Geometry: final body of the model. Coordinates: model frame, mm. Give positions to 0.01 mm unless a question says otherwise; leave off trailing zeros. Write each loop counter-clockwise with the first axis right and the second up, starting at its lowest first coordinate (ties: lowest second). Pieces come first, ordered by that corner, then holes.
Q1. Draft query along Y for faces 1 (the face through (230.495, 14.758, 19.367)), 2 (the face through (0, 67, 20)), 3 (the face through (4.51, 4.28, 19.72)), 4 (the face through (210.974, 29.257, 24.79)). Return one class per face: pulls with the +Y half, pulls with the -Y half, needs draft (parallel to the pull), parting line crosses it, or undercut.
Q2. Pin query (flat end, axial travel): pin 1 (5.5 mm diameter, centred on x = 226, y = 15, fed in from +Z); pin 2 (9 mm diameter, centred on x = 224, y = 121, fed in from +Z); pin 3 (4.5 mm diameter, centred on x = 160, y = 73.79, fed in from +Z). Return the tip coordinate at first contact, or that it passes through.
Q3. Cut plane B-B on z = 22. Count the separate pieces of the cut face and the enclosed holes in it, plus the area to 3 significant figures.
Q4. Cut plane A-A on y = 43.5. Return the cut outline in (x, z).
Q5. Line query: L1, parallel to X at y = 78, z = 11; L2, parallel to Y at x = 80, z = 26.25; L3, parallel to Y at x = 40.5, z = 30. Output: solid intervals per line, ascending.
```python
from build123d import *

# Parameters (mm, degrees)
SKETCH_1_R                   = 5.5
EXTRUDE_1_DEPTH              = 40
EXTRUDE_2_DEPTH              = 10
EXTRUDE_3_DEPTH              = 20
HOLE_WIZARD_M6_3_D           = 5
HOLE_WIZARD_M6_3_DEPTH       = 15
HOLE_WIZARD_M6_3_CSINK_D     = 8
HOLE_WIZARD_M6_3_CSINK_ANGLE = 90
HOLE_WIZARD_M6_3_TIP         = 1.502151548
SKETCH_9_R                   = 9
CUT_EXTRUDE_1_DEPTH          = 11
CHAMFER_2_SIZE               = 1
CHAMFER_3_SIZE               = 1


with BuildPart() as part:
    # 草图1 → 凸台-拉伸1 (new body)
    with BuildSketch(Plane.XY):
        with BuildLine():
            Line((0, 15), (0, 120))
            ThreePointArc((0, 120), (4.393398282, 130.606601718), (15, 135))
            Line((15, 135), (225, 135))
            ThreePointArc((225, 135), (235.606601718, 130.606601718), (240, 120))
            Line((240, 120), (240, 15))
            ThreePointArc((240, 15), (235.606601718, 4.393398282), (225, 0))
            Line((225, 0), (15, 0))
            ThreePointArc((15, 0), (4.393398282, 4.393398282), (0, 15))
        make_face()
        with Locations((225, 120)):
            Circle(SKETCH_1_R, mode=Mode.SUBTRACT)
        with Locations(Location((225, 15, 0), (0, 0, 180))):
            Circle(SKETCH_1_R, mode=Mode.SUBTRACT)
        with Locations((15, 15)):
            Circle(SKETCH_1_R, mode=Mode.SUBTRACT)
        with Locations(Location((15, 120, 0), (0, 0, 180))):
            Circle(SKETCH_1_R, mode=Mode.SUBTRACT)
        with BuildLine():
            Line((15, 39.494897428), (15, 95.505102572))
            ThreePointArc((15, 95.505102572), (16.127016654, 98.667380232), (19, 100.404082058))
            ThreePointArc((19, 100.404082058), (29.142135624, 105.857864376), (34.595917942, 116))
            ThreePointArc((34.595917942, 116), (36.332619768, 118.872983346), (39.494897428, 120))
            Line((39.494897428, 120), (200.505102572, 120))
            ThreePointArc((200.505102572, 120), (203.667380232, 118.872983346), (205.404082058, 116))
            ThreePointArc((205.404082058, 116), (210.857864376, 105.857864376), (221, 100.404082058))
            ThreePointArc((221, 100.404082058), (223.872983346, 98.667380232), (225, 95.505102572))
            Line((225, 95.505102572), (225, 39.494897428))
            ThreePointArc((225, 39.494897428), (223.872983346, 36.332619768), (221, 34.595917942))
            ThreePointArc((221, 34.595917942), (210.857864376, 29.142135624), (205.404082058, 19))
            ThreePointArc((205.404082058, 19), (203.667380232, 16.127016654), (200.505102572, 15))
            Line((200.505102572, 15), (39.494897428, 15))
            ThreePointArc((39.494897428, 15), (36.332619768, 16.127016654), (34.595917942, 19))
            ThreePointArc((34.595917942, 19), (29.142135624, 29.142135624), (19, 34.595917942))
            ThreePointArc((19, 34.595917942), (16.127016654, 36.332619768), (15, 39.494897428))
        make_face(mode=Mode.SUBTRACT)
    extrude(amount=EXTRUDE_1_DEPTH)

    # 草图2 → 凸台-拉伸2 (add)
    with BuildSketch(Plane(origin=(0, 0, 0), x_dir=(-1, 0, 0), z_dir=(0, 0, -1))):
        with BuildLine():
            Line((-225, 135), (-15, 135))
            ThreePointArc((-15, 135), (-4.393398282, 130.606601718), (0, 120))
            Line((0, 120), (0, 15))
            ThreePointArc((0, 15), (-4.393398282, 4.393398282), (-15, 0))
            Line((-15, 0), (-225, 0))
            ThreePointArc((-225, 0), (-235.606601718, 4.393398282), (-240, 15))
            Line((-240, 15), (-240, 120))
            ThreePointArc((-240, 120), (-235.606601718, 130.606601718), (-225, 135))
        make_face()
    extrude(amount=-EXTRUDE_2_DEPTH)

    # 草图3 → 凸台-拉伸3 (add)
    with BuildSketch(Plane.XY.offset(10)):
        with BuildLine():
            Line((72, 81.293943495), (168, 81.293943495))
            ThreePointArc((168, 81.293943495), (169.414213562, 80.708157058), (170, 79.293943495))
            Line((170, 79.293943495), (170, 53.293943495))
            ThreePointArc((170, 53.293943495), (169.414213562, 51.879729933), (168, 51.293943495))
            Line((168, 51.293943495), (156.201767504, 51.293943495))
            ThreePointArc((156.201767504, 51.293943495), (155.208790822, 51.557856715), (154.477873813, 52.279946186))
            ThreePointArc((154.477873813, 52.279946186), (120, 72), (85.522126187, 52.279946186))
            ThreePointArc((85.522126187, 52.279946186), (84.791209178, 51.557856715), (83.798232496, 51.293943495))
            Line((83.798232496, 51.293943495), (72, 51.293943495))
            ThreePointArc((72, 51.293943495), (70.585786438, 51.879729933), (70, 53.293943495))
            Line((70, 53.293943495), (70, 79.293943495))
            ThreePointArc((70, 79.293943495), (70.585786438, 80.708157058), (72, 81.293943495))
        make_face()
    extrude(amount=EXTRUDE_3_DEPTH)

    # M6 螺纹孔3
    with Locations(Plane(origin=(80, 73.793943495, 30), x_dir=(1, 0, 0), z_dir=(0, 0, 1))):
        with Locations((0, 0), (0, -12.58788699), (80, 0), (80, -12.58788699)):
            CounterSinkHole(HOLE_WIZARD_M6_3_D / 2, HOLE_WIZARD_M6_3_CSINK_D / 2, depth=HOLE_WIZARD_M6_3_DEPTH, counter_sink_angle=HOLE_WIZARD_M6_3_CSINK_ANGLE)
            with Locations((0, 0, -(HOLE_WIZARD_M6_3_DEPTH + HOLE_WIZARD_M6_3_TIP / 2))):  # 118° drill point
                Cone(0, HOLE_WIZARD_M6_3_D / 2, HOLE_WIZARD_M6_3_TIP, mode=Mode.SUBTRACT)

    # 草图9 → 切除-拉伸1 (cut)
    with BuildSketch(Plane.XY.offset(40)):
        with Locations((15, 120)):
            Circle(SKETCH_9_R)
        with Locations((15, 15)):
            Circle(SKETCH_9_R)
        with Locations((225, 120)):
            Circle(SKETCH_9_R)
        with Locations((225, 15)):
            Circle(SKETCH_9_R)
    extrude(amount=-CUT_EXTRUDE_1_DEPTH, mode=Mode.SUBTRACT)

    # 倒角2
    chamfer_2_edges = [part.edges().sort_by_distance(p)[0] for p in [
        (6, 15, 40),
        (216, 120, 40),
        (216, 15, 40),
        (6, 120, 40),
    ]]
    chamfer(chamfer_2_edges, length=CHAMFER_2_SIZE)

    # 倒角3
    chamfer_3_edges = [part.edges().sort_by_distance(p)[0] for p in [
        (70.585786438, 51.879729933, 30),
        (155.208790822, 51.557856715, 30),
        (162.100883752, 51.293943495, 30),
        (169.414213562, 51.879729933, 30),
        (170, 66.293943495, 30),
        (169.414213562, 80.708157058, 30),
        (120, 81.293943495, 30),
        (70.585786438, 80.708157058, 30),
        (70, 66.293943495, 30),
        (77.899116248, 51.293943495, 30),
        (84.791209178, 51.557856715, 30),
        (120, 72, 30),
    ]]
    chamfer(chamfer_3_edges, length=CHAMFER_3_SIZE)


solid = part.part
```
Data:
1. face 1: undercut
1. face 2: needs draft
1. face 3: pulls with the -Y half
1. face 4: undercut
2. pin 1: stops at z = 10
2. pin 2: stops at z = 29
2. pin 3: stops at z = 14.85
3. separate pieces: 2
3. enclosed holes: 9
3. area: 12,900 mm2
4. outline: (0, 0) - (240, 0) - (240, 40) - (225, 40) - (225, 10) - (15, 10) - (15, 40) - (0, 40) - close
5. L1: x = 0 to 15, 70 to 170, 225 to 240
5. L2: y = 0 to 15, 51.29 to 58.71, 63.71 to 71.29, 76.29 to 81.29, 120 to 135
5. L3: y = 0 to 15, 120 to 135
